The listing builds one solid part. Answer for the finished solid, in the listing's coordinates (mm). Face numbers are marked on the shaded views. A direction names the side the tool comes from. Round coordinates to 2 decimals unless told otherwise and drop trailing zeros. Order: outer loops, then holes, each group sorted by start corner. A loop starts at its lowest first (then second) coordinate and runs counter-clockwise, first axis right, second up. Notation, with made-up numbers: (-6.75, 47) -> (45.25, 47) arc R14 cw to (45.25, 71) -> close; hole circle Ø9 at (-14.5, 27). An arc over 180 degrees is marked (long way). Return JSON: item names as keys, results as strings. Group by question number.
(1) The part is cut by section D-D (x = -36). Determine the outline of the cut face in (y, z) (3 decimals).
(2) Each of these flat-tipped pins is pushed along its axis until it touches: pin 1 (10.5 mm diameter, centred on x = -19.05, z = -5.08, fed in from +Y); pin 2 (10 mm diameter, centred on x = -28.5, z = -34.5, fed in from +Y); pin 3 (1 mm diameter, centred on x = -21.5, z = -17, fed in from +Y); pin 4 (12.5 mm diameter, centred on x = 9, y = -15, fed in from +Z). Where does it stop, or does it pass through?
(3) Which of the six approach directions +Z, -Z, +X, -X, +Y, -Y give full straight-line access (tool end or side, diameter ignored) to the marked faces 1 and 2?
(4) The part is cut by section B-B (z = -40.5). Determine the outline of the cut face in (x, y) (3 decimals), plus the area to 3 significant figures.
(5) Consider line 1 (X direction, y = -52.6, z = -5.08); line 2 (Y direction, x = 0, z = -45.5) (3 decimals); line 3 (X direction, y = -11, z = -15). Determine where each line is inside the solid, lowest interval first. Write a range as [from, to].
(6) Determine the mould class of the marked faces 3, 4, 5 and 6 for opening direction Y: +Y half, -Y half, draft (parallel to the pull), parting line (faces both ways), or undercut.
(7) The part is cut by section C-C (z = -50.8). Count the separate pieces of the cut face and the enclosed holes in it, plus the area to 3 significant figures.
(8) The part is cut by section A-A (y = -10). Determine the outline of the cut face in (x, z) (3 decimals), plus the area to 3 significant figures.
from build123d import *

# Parameters (mm, degrees)
BOSS_EXTRUDE2_DEPTH = 12.7
CUT_EXTRUDE1_DEPTH  = 12.7
CUT_EXTRUDE2_START  = -12.7
CUT_EXTRUDE2_DEPTH  = 12.7
BOSS_EXTRUDE3_REACH = 106.45
SKETCH9_R           = 3.3020000000000005
SKETCH9_R_2         = 3.3019999999999987
CUT_EXTRUDE3_DEPTH  = 93.09259864397356
CUT_EXTRUDE4_START  = -3.175
CUT_EXTRUDE4_DEPTH  = 6.8580000000000005
BOSS_EXTRUDE6_DEPTH = 38.1
SKETCH12_W          = 25.4
SKETCH12_H          = 6.350000000000001
BOSS_EXTRUDE4_DEPTH = 25.4
CUT_EXTRUDE5_START  = 39.370000000000005
CUT_EXTRUDE5_DEPTH  = 6.8580000000000005
SKETCH13_R          = 3.302000000000001
CUT_EXTRUDE6_DEPTH  = 93.09259864397356
CIRPATTERN1_COUNT   = 4
BOSS_EXTRUDE5_START = 38.1
BOSS_EXTRUDE5_DEPTH = 38.1
SKETCH16_W          = 3.1749999999999687
SKETCH16_H          = 40.98999999999984
SKETCH16_W_2        = 3.1750000000001393
SKETCH16_H_2        = 40.990000000000464
BOSS_EXTRUDE7_DEPTH = 63.5
BOSS_EXTRUDE9_START = -63.5
BOSS_EXTRUDE9_DEPTH = 63.5


with BuildPart() as part:
    # Sketch2 → Revolve1 (revolve)
    with BuildSketch(Plane(origin=(0, 0, 0), x_dir=(1, 0, 0), z_dir=(0, 1, 0))):
        Polygon((25.75, 0), (25.75, 2.14), (26.874999999999996, 5.319999999999995), (26.874999999999993, 25.400000000000006), (39.574999999999996, 25.400000000000002), (39.574999999999974, 5.62e-15), align=None)
    revolve(axis=Axis((0, 0, 0), (0, 0, -1)))

    # Sketch3 → Boss-Extrude2 (add)
    with BuildSketch(Plane.XY):
        Polygon((26.87499999999997, 0), (39.574999999999974, 0), (39.57499999999997, -53.690000000000005), (-39.57499999999997, -53.690000000000005), (-39.574999999999974, 0), (-26.874999999999975, 0), (-26.874999999999968, -40.99), (26.874999999999975, -40.99), align=None)
    extrude(amount=-BOSS_EXTRUDE2_DEPTH)

    # Sketch5 → Cut-Extrude1 (cut)
    with BuildSketch(Plane.XY):
        Polygon((26.874999999999975, -40.99), (-26.874999999999968, -40.99000000000001), (-26.874999999999968, -6.94e-15), (26.874999999999975, -7.8e-16), align=None)
    extrude(amount=-CUT_EXTRUDE1_DEPTH, mode=Mode.SUBTRACT)

    # Sketch6 → Cut-Extrude2 (cut)
    with BuildSketch(Plane.XY.offset(CUT_EXTRUDE2_START)):
        with BuildLine():
            Line((-22.832761550018414, 14.174999999999976), (22.832761550018414, 14.174999999999976))
            ThreePointArc((22.832761550018414, 14.174999999999976), (-4.94e-15, -26.874999999999975), (-22.832761550018414, 14.174999999999976))
        make_face()
    extrude(amount=CUT_EXTRUDE2_DEPTH, mode=Mode.SUBTRACT)

    # Sketch7 → Boss-Extrude3 (add, up to next)
    with BuildSketch(Plane.XZ.offset(53.690000000000005), mode=Mode.PRIVATE) as boss_extrude3_sk1:
        Polygon((39.57499999999997, -12.7), (-39.57499999999997, -12.70000000000001), (-39.57499999999997, -25.40000000000001), (39.57499999999997, -25.4), align=None)
    boss_extrude3_tool1 = extrude(boss_extrude3_sk1.sketch, amount=-BOSS_EXTRUDE3_REACH, mode=Mode.PRIVATE) - part.part
    add(boss_extrude3_tool1.solids().sort_by_distance((0, -53.69, -19.05))[0])

    # Sketch8 → Revolve2 (revolve)
    with BuildSketch(Plane(origin=(0, 0, 0), x_dir=(1, 0, 0), z_dir=(0, 1, 0)), mode=Mode.PRIVATE) as revolve2_sk:
        Polygon((-39.574999999999996, 25.400000000000002), (-39.574999999999974, 63.5), (-29.844999999999995, 63.5), (-29.844999999999995, 25.400000000000006), align=None)
    revolve(revolve2_sk.sketch.rotate(Axis((0, 0, -2.42e-15), (0, 0, -1)), 180), axis=Axis((0, 0, -2.42e-15), (0, 0, -1)))

    # Sketch9 → Cut-Extrude3 (cut, through all)
    with BuildSketch(Plane(origin=(0, 0, 0), x_dir=(1, 0, 0), z_dir=(0, 1, 0))):
        with Locations(Location((0, 5.08, 0), (0, 0, 270))):
            Circle(SKETCH9_R)
        with Locations(Location((19.05, 5.080000000000001, 0), (0, 0, 270))):
            Circle(SKETCH9_R_2)
        with Locations(Location((-19.05, 5.08, 0), (0, 0, 270))):
            Circle(SKETCH9_R_2)
    extrude(amount=-CUT_EXTRUDE3_DEPTH, mode=Mode.SUBTRACT)

    # Sketch10 → Cut-Extrude4 (cut)
    with BuildSketch(Plane(origin=(0, -53.690000000000005, 0), x_dir=(-1, 0, 0), z_dir=(0, -1, 0)).offset(CUT_EXTRUDE4_START)):
        Polygon((-24.511, 1.927090179955452), (-24.765, -8.7e-16), (-13.334999999999999, -8.7e-16), (-13.589, 1.927090179955445), (-13.589, 8.232909820044544), (-19.050000000000004, 11.385819640089089), (-24.511, 8.232909820044545), align=None)
        Polygon((1.88e-15, 11.385819640089093), (-5.460999999999999, 8.232909820044547), (-5.461, 1.9270901799554545), (-5.715, 0), (5.715, 0), (5.4609999999999985, 1.9270901799554514), (5.4609999999999985, 8.232909820044547), align=None)
        Polygon((19.049999999999997, 11.385819640089094), (13.589, 8.23290982004455), (13.589, 1.9270901799554547), (13.335, 8.7e-16), (24.765, 8.7e-16), (24.511000000000003, 1.9270901799554534), (24.511, 8.232909820044547), align=None)
    extrude(amount=-CUT_EXTRUDE4_DEPTH, mode=Mode.SUBTRACT)

    # Sketch15 → Boss-Extrude6 (add)
    with BuildSketch(Plane(origin=(0, 0, -25.400000000000006), x_dir=(-1, 0, 0), z_dir=(0, 0, -1))):
        with BuildLine():
            Line((39.57499999999997, -53.690000000000005), (39.574999999999996, 0))
            ThreePointArc((39.574999999999996, 0), (-7.27e-15, -39.574999999999996), (-39.574999999999996, 4.85e-15))
            Line((-39.574999999999996, 4.85e-15), (-39.57499999999997, -53.690000000000005))
            Line((-39.57499999999997, -53.690000000000005), (39.57499999999997, -53.690000000000005))
        make_face()
    extrude(amount=BOSS_EXTRUDE6_DEPTH)

    # Sketch12 → Boss-Extrude4 (add)
    with BuildSketch(Plane(origin=(0, 0, -63.5), x_dir=(-1, 0, 0), z_dir=(0, 0, -1))):
        with Locations((1.155e-14, 39.574999999999974)):
            Rectangle(SKETCH12_W, SKETCH12_H)
    boss_extrude4 = extrude(amount=-BOSS_EXTRUDE4_DEPTH)

    # Sketch11 → Cut-Extrude5 (cut)
    with BuildSketch(Plane(origin=(0, 0, 0), x_dir=(1, 0, 0), z_dir=(0, 1, 0)).offset(CUT_EXTRUDE5_START)):
        Polygon((-6.92e-15, 44.4941803599109), (5.460999999999995, 47.64709017995545), (5.460999999999995, 53.95290982004454), (5.715, 63.5), (-5.715, 63.5), (-5.461000000000004, 53.95290982004454), (-5.461000000000002, 47.64709017995544), align=None)
    cut_extrude5 = extrude(amount=-CUT_EXTRUDE5_DEPTH, mode=Mode.SUBTRACT)

    # Sketch13 → Cut-Extrude6 (cut, through all)
    with BuildSketch(Plane(origin=(0, 0, 0), x_dir=(1, 0, 0), z_dir=(0, 1, 0))):
        with Locations(Location((0, 50.8, 0), (0, 0, 90))):
            Circle(SKETCH13_R)
    cut_extrude6 = extrude(amount=CUT_EXTRUDE6_DEPTH, mode=Mode.SUBTRACT)

    # CirPattern1: Boss-Extrude4, Cut-Extrude5, Cut-Extrude6 ×4 about axis
    cirpattern1_axis = Axis((-1.2e-16, 3e-17, 0), (0, 0, 1))
    add([boss_extrude4.rotate(cirpattern1_axis, i * 360 / CIRPATTERN1_COUNT) for i in range(1, CIRPATTERN1_COUNT)])
    add([cut_extrude5.rotate(cirpattern1_axis, i * 360 / CIRPATTERN1_COUNT) for i in range(1, CIRPATTERN1_COUNT)], mode=Mode.SUBTRACT)
    add([cut_extrude6.rotate(cirpattern1_axis, i * 360 / CIRPATTERN1_COUNT) for i in range(1, CIRPATTERN1_COUNT)], mode=Mode.SUBTRACT)

    # Sketch14 → Boss-Extrude5 (add)
    with BuildSketch(Plane.XY.offset(-38.1).offset(BOSS_EXTRUDE5_START)):
        with BuildLine():
            Line((39.574999999999974, -12.699999999999605), (42.75000000000011, -12.69999999999954))
            Line((42.75000000000011, -12.69999999999954), (42.749999999999844, 12.70000000000046))
            Line((42.749999999999844, 12.70000000000046), (37.48187061767313, 12.7000000000004))
            ThreePointArc((37.48187061767313, 12.7000000000004), (39.048211576808555, 6.435666061317394), (39.57499999999998, 0))
            Line((39.57499999999998, 0), (39.574999999999974, -12.699999999999605))
        make_face()
        with BuildLine():
            Line((12.699999999999985, 37.48187061767327), (12.699999999999987, 42.74999999999998))
            Line((12.699999999999987, 42.74999999999998), (-12.700000000000012, 42.74999999999998))
            Line((-12.700000000000012, 42.74999999999998), (-12.700000000000014, 37.481870617673266))
            ThreePointArc((-12.700000000000014, 37.481870617673266), (-1.515e-14, 39.57499999999998), (12.699999999999985, 37.48187061767327))
        make_face()
        with BuildLine():
            Line((-37.48187061767331, 12.699999999999852), (-42.750000000000014, 12.699999999999838))
            Line((-42.750000000000014, 12.699999999999838), (-42.749999999999936, -12.700000000000161))
            Line((-42.749999999999936, -12.700000000000161), (-39.574999999999974, -12.700000000000161))
            Line((-39.574999999999974, -12.700000000000161), (-39.57499999999998, 4.85e-15))
            ThreePointArc((-39.57499999999998, 4.85e-15), (-39.0482115768086, 6.435666061317119), (-37.48187061767331, 12.699999999999852))
        make_face()
    extrude(amount=-BOSS_EXTRUDE5_DEPTH)

    # Sketch16 → Boss-Extrude7 (add)
    with BuildSketch(Plane(origin=(0, 0, -63.5), x_dir=(-1, 0, 0), z_dir=(0, 0, -1))):
        with Locations((41.16249999999995, -33.195000000000086)):
            Rectangle(SKETCH16_W, SKETCH16_H)
        with Locations((-41.16250000000004, -33.19499999999977)):
            Rectangle(SKETCH16_W_2, SKETCH16_H_2)
    extrude(amount=-BOSS_EXTRUDE7_DEPTH)

    # Sketch17 → Boss-Extrude9 (add)
    with BuildSketch(Plane(origin=(0, 0, -63.5), x_dir=(-1, 0, 0), z_dir=(0, 0, -1)).offset(BOSS_EXTRUDE9_START)):
        with BuildLine():
            Line((-42.749999999999844, 12.70000000000046), (-37.481870617673124, 12.700000000000404))
            ThreePointArc((-37.481870617673124, 12.700000000000404), (-27.98375086545744, 27.983750865457754), (-12.699999999999989, 37.48187061767326))
            Line((-12.699999999999989, 37.48187061767326), (-12.699999999999987, 42.74999999999998))
            ThreePointArc((-12.699999999999987, 42.74999999999998), (-31.53452473084045, 31.534524730840808), (-42.749999999999844, 12.70000000000046))
        make_face()
        with BuildLine():
            Line((37.481870617673124, 12.700000000000404), (42.750000000000014, 12.699999999999838))
            ThreePointArc((42.750000000000014, 12.699999999999838), (31.534524730840676, 31.53452473084055), (12.700000000000012, 42.74999999999998))
            Line((12.700000000000012, 42.74999999999998), (12.700000000000012, 37.48187061767325))
            ThreePointArc((12.700000000000012, 37.48187061767325), (27.98375086545745, 27.983750865457747), (37.481870617673124, 12.700000000000404))
        make_face()
    extrude(amount=BOSS_EXTRUDE9_DEPTH)


solid = part.part
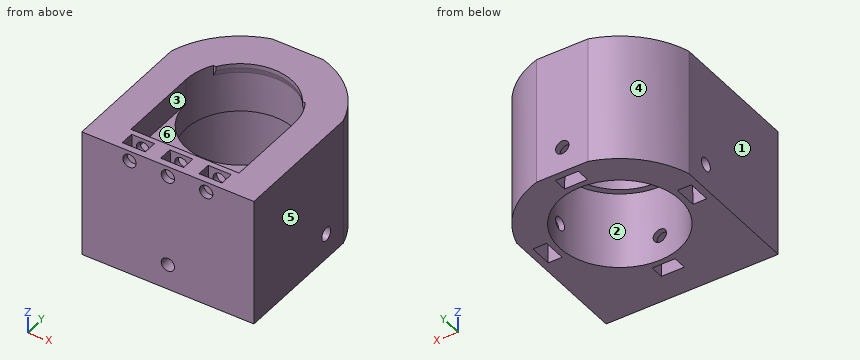
Answer below:
{
 "1": {"outline": "(-53.69, -63.5) -> (-5.715, -63.5) -> (-5.461, -53.953) -> (-5.461, -47.647) -> (0, -44.494) -> (5.461, -47.647) -> (5.461, -53.953) -> (5.715, -63.5) -> (26.322, -63.5) -> (26.322, 0) -> (-53.69, 0) -> close"},
 "2": {"pin 1": "stops at y = 42.41", "pin 2": "stops at y = 37.9", "pin 3": "stops at y = 39.34", "pin 4": "passes through"},
 "3": {"face 1": "+Z, -Z, -X, +Y, -Y", "face 2": "-Z"},
 "4": {"outline": "(-42.75, -53.69) -> (42.75, -53.69) -> (42.75, 12.7) arc R44.597 ccw to (12.7, 42.75) -> (-12.7, 42.75) arc R44.597 ccw to (-42.75, 12.7) -> close; hole circle Ø59.69 at (0, 0)", "area": "4,850 mm²"},
 "5": {"line 1": "x = [-42.75, -22.35], [-15.75, -3.3], [3.3, 15.75], [22.35, 42.75]", "line 2": "y = [-53.69, -39.37], [-32.512, -29.845], [29.845, 32.512], [39.37, 42.75]", "line 3": "x = [-42.75, -24.52], [24.52, 42.75]"},
 "6": {"face 3": "undercut", "face 4": "+Y half", "face 5": "draft", "face 6": "undercut"},
 "7": {"separate pieces": "4", "enclosed holes": "0", "area": "4,320 mm²"},
 "8": {"outline": "(-42.75, -63.5) -> (-28.12, -63.5) -> (-28.12, -25.4) -> (-24.945, -25.4) -> (-24.945, -12.7) -> (-26.875, -12.7) -> (-26.875, 0) -> (-42.75, 0) -> close; (24.945, -25.4) -> (28.12, -25.4) -> (28.12, -63.5) -> (42.75, -63.5) -> (42.75, 0) -> (26.875, 0) -> (26.875, -12.7) -> (24.945, -12.7) -> close", "area": "1,970 mm²"}
}
